Geometry check sheet. Reference: the model listing, model coordinates, mm. Give positions to 0.01 mm unless a question says otherwise; leave off trailing zeros. Write each loop counter-clockwise with the first axis right and the second up, starting at its lowest first coordinate (ties: lowest second). Pieces come first, ordered by that corner, then holes. Notation, with made-up numbers: (85.25, 73) -> (112.25, 73) arc R13 ccw to (112.25, 87) -> close; hole circle Ø5 at (49.5, 72). An arc over 180 degrees is marked (long way). Use a Markdown table: item, result. Add a question column.
from build123d import *

# Parameters (mm, degrees)
BOSS_EXTRUDE1_DEPTH                  = 7.9248
SKETCH12_W                           = 35.56
SKETCH12_H                           = 35.56
FILLET1_R                            = 1.016
F_8_32_TAPPED_HOLE2_AT_2_COUNT       = 2
F_8_32_TAPPED_HOLE2_AT_2_PITCH       = 19.05
F_8_32_TAPPED_HOLE2_AT_3_COUNT       = 2
F_8_32_TAPPED_HOLE2_AT_3_PITCH       = 117.4496
F_8_32_TAPPED_HOLE2_AT_4_COUNT       = 2
F_8_32_TAPPED_HOLE2_AT_4_PITCH       = 118.984499159
F_17_0_173_DIAMETER_HOLE1_AT_2_COUNT = 2
F_17_0_173_DIAMETER_HOLE1_AT_2_PITCH = 19.05
F_17_0_173_DIAMETER_HOLE1_AT_3_COUNT = 2
F_17_0_173_DIAMETER_HOLE1_AT_3_PITCH = 139.7
F_17_0_173_DIAMETER_HOLE1_AT_4_COUNT = 2
F_17_0_173_DIAMETER_HOLE1_AT_4_PITCH = 140.992881026


with BuildPart() as part:
    # Sketch1 → Boss-Extrude1 (new body)
    with BuildSketch(Plane(origin=(0, 0, 0), x_dir=(1, 0, 0), z_dir=(0, 0, -1))):
        with BuildLine():
            Line((74.008534906, -15.875), (-74.008534906, -15.875))
            ThreePointArc((-74.008534906, -15.875), (-75.692, 0), (-74.008534906, 15.875))
            Line((-74.008534906, 15.875), (74.008534906, 15.875))
            ThreePointArc((74.008534906, 15.875), (75.692, 0), (74.008534906, -15.875))
        make_face()
    extrude(amount=-BOSS_EXTRUDE1_DEPTH)

    # Sketch12 → Cut-Revolve1 (revolve, cut)
    with BuildSketch(Plane(origin=(0, 0, 0), x_dir=(1, 0, 0), z_dir=(0, 1, 0))):
        with Locations((82.6008, 16.764)):
            Rectangle(SKETCH12_W, SKETCH12_H)
    revolve(axis=Axis((0, 0, -12.484857721), (0, 0, -1)), mode=Mode.SUBTRACT)

    # Fillet1
    fillet1_edges = [part.edges().sort_by_distance(p)[0] for p in [
        (74.008534906, 15.875, 4.4704),
        (-74.008534906, 15.875, 4.4704),
        (-74.008534906, -15.875, 4.4704),
        (74.008534906, -15.875, 4.4704),
    ]]
    fillet(fillet1_edges, radius=FILLET1_R)

    # Sketch2 → #8-32 Tapped Hole2 (revolve, cut)
    with BuildSketch(Plane(origin=(-58.7248, 9.525, 0), x_dir=(0, 1, 0), z_dir=(1, 0, 0))):
        Polygon((0, 0), (0, 7.9248), (3.048, 7.9248), (1.7272, 6.604), (1.7272, 0.5588), (2.286, 0), align=None)
    f_8_32_tapped_hole2 = revolve(axis=Axis((-58.7248, 9.525, -6.35), (0, 0, 1)), mode=Mode.SUBTRACT)

    # #8-32 Tapped Hole2 at 2: #8-32 Tapped Hole2 ×2
    with Locations(*[(0, -i * F_8_32_TAPPED_HOLE2_AT_2_PITCH, 0) for i in range(1, F_8_32_TAPPED_HOLE2_AT_2_COUNT)]):
        add(f_8_32_tapped_hole2, mode=Mode.SUBTRACT)

    # #8-32 Tapped Hole2 at 3: #8-32 Tapped Hole2 ×2
    with Locations(*[(i * F_8_32_TAPPED_HOLE2_AT_3_PITCH, 0, 0) for i in range(1, F_8_32_TAPPED_HOLE2_AT_3_COUNT)]):
        add(f_8_32_tapped_hole2, mode=Mode.SUBTRACT)

    # #8-32 Tapped Hole2 at 4: #8-32 Tapped Hole2 ×2
    with Locations(*[Vector(0.9871000073957296, -0.16010488874281947, 0) * (i * F_8_32_TAPPED_HOLE2_AT_4_PITCH) for i in range(1, F_8_32_TAPPED_HOLE2_AT_4_COUNT)]):
        add(f_8_32_tapped_hole2, mode=Mode.SUBTRACT)

    # Sketch5 → #17 (0.173) Diameter Hole1 (revolve, cut)
    with BuildSketch(Plane(origin=(69.85, 9.525, 7.9248), x_dir=(0, -1, 0), z_dir=(1, 0, 0))):
        Polygon((0, 0), (0, 6.9088), (2.4892, 6.9088), (2.1971, 6.6167), (2.1971, 0.2921), (2.4892, 0), align=None)
    f_17_0_173_diameter_hole1 = revolve(axis=Axis((69.85, 9.525, 14.2748), (0, 0, -1)), mode=Mode.SUBTRACT)

    # #17 (0.173) Diameter Hole1 at 2: #17 (0.173) Diameter Hole1 ×2
    with Locations(*[(0, -i * F_17_0_173_DIAMETER_HOLE1_AT_2_PITCH, 0) for i in range(1, F_17_0_173_DIAMETER_HOLE1_AT_2_COUNT)]):
        add(f_17_0_173_diameter_hole1, mode=Mode.SUBTRACT)

    # #17 (0.173) Diameter Hole1 at 3: #17 (0.173) Diameter Hole1 ×2
    with Locations(*[(-i * F_17_0_173_DIAMETER_HOLE1_AT_3_PITCH, 0, 0) for i in range(1, F_17_0_173_DIAMETER_HOLE1_AT_3_COUNT)]):
        add(f_17_0_173_diameter_hole1, mode=Mode.SUBTRACT)

    # #17 (0.173) Diameter Hole1 at 4: #17 (0.173) Diameter Hole1 ×2
    with Locations(*[Vector(-0.990830168044299, -0.13511320473331354, 0) * (i * F_17_0_173_DIAMETER_HOLE1_AT_4_PITCH) for i in range(1, F_17_0_173_DIAMETER_HOLE1_AT_4_COUNT)]):
        add(f_17_0_173_diameter_hole1, mode=Mode.SUBTRACT)


solid = part.part
1) Draft check along X on faces 1 (the face through (1, 0, 0)), 2 (the face through (71.995, -9.049, 4.515)). Enter one of: +X half, -X half, draft (parallel to the pull), parting line (faces both ways), or undercut.
2) Gauge pin test, flat ends, axial feed: P1, Ø7, axis at x = 69.85, y = -9.525, coming from the -Z side; P2, Ø4, axis at y = 12.5, z = 4.5, coming from the -X side. Record the tip position at first contact, or that the pin passes through.
3) Material ranges on probe 1 along Y at (x, z) = (-69.85, 3.25) (3 decimals); probe 2 along X at (y, z) = (11, 1.25); probe 3 along X at (y, z) = (11, 4.75), recorded low to high. Write a range as [from, to].
4) Sectioned sample at A-A, the plane x = -69.85. Enter the section's corners in (y, z) (3 decimals).
5) Sectioned sample at C-C, the plane y = -4. Enter the section's corners in (x, z).
6) Sectioned sample at B-B, the plane z = 5. Count the separate pieces of the cut face and the enclosed holes in it, and give its area (3 significant figures).
Check values:
| question | item | result |
|---|---|---|
| 1 | face 1 | draft |
| 1 | face 2 | undercut |
| 2 | P1 | z = 1.02 |
| 2 | P2 | x = -74.96 |
| 3 | probe 1 | [-15.875, -11.722], [-7.328, 7.328], [11.722, 15.875] |
| 3 | probe 2 | [-74.89, -71.56], [-68.14, -59.62], [-57.83, 57.83], [59.62, 68.14], [71.56, 74.89] |
| 3 | probe 3 | [-74.89, -71.48], [-68.22, -59.62], [-57.83, 57.83], [59.62, 68.22], [71.48, 74.89] |
| 4 | outline | (-15.875, 1.016) -> (-12.014, 1.016) -> (-11.722, 1.308) -> (-11.722, 7.633) -> (-12.014, 7.925) -> (-15.875, 7.925) -> close; (-7.328, 1.308) -> (-7.036, 1.016) -> (7.036, 1.016) -> (7.328, 1.308) -> (7.328, 7.633) -> (7.036, 7.925) -> (-7.036, 7.925) -> (-7.328, 7.633) -> close; (11.722, 1.308) -> (12.014, 1.016) -> (15.875, 1.016) -> (15.875, 7.925) -> (12.014, 7.925) -> (11.722, 7.633) -> close |
| 5 | outline | (-75.59, 1.02) -> (-64.7, 1.02) -> (-64.7, 0) -> (64.7, 0) -> (64.7, 1.02) -> (75.59, 1.02) -> (75.59, 7.92) -> (-75.59, 7.92) -> close |
| 6 | separate pieces | 1 |
| 6 | enclosed holes | 8 |
| 6 | area | 4,670 mm² |
